Source: CAD feature listing. Evaluate the final solid. Frame: model axes, mm. Face numbers are marked on the shaded views. A direction names the side the tool comes from. Coordinates: 2 decimals unless noted, no trailing zeros. Order: outer loops, then holes, each group sorted by start corner. A loop starts at its lowest first (then second) coordinate and runs counter-clockwise, first axis right, second up.
```python
from build123d import *

# Parameters (mm, degrees)
SKETCH_1_W          = 15
SKETCH_1_H          = 10
EXTRUDE_1_DEPTH     = 5
SKETCH_1_3_W        = 15
SKETCH_1_3_H        = 10
EXTRUDE_2_DEPTH     = 15
CUT_EXTRUDE_1_DEPTH = 15


with BuildPart() as part:
    # Sketch 1 → Extrude 1 (new body)
    with BuildSketch(Plane(origin=(0, 0, 0), x_dir=(1, 0, 0), z_dir=(0, 1, 0))):
        Polygon((-5, -10), (0, -10), (15, 10), (0, 10), (0, 0), (-15, 0), (-15, -5), (-5, -5), align=None)
        with Locations((-7.5, 5)):
            Rectangle(SKETCH_1_W, SKETCH_1_H)
    extrude(amount=EXTRUDE_1_DEPTH)

    # Sketch 1_3 → Extrude 2 (add)
    with BuildSketch(Plane(origin=(0, 0, 0), x_dir=(1, 0, 0), z_dir=(0, 1, 0))):
        with Locations((-7.5, 5)):
            Rectangle(SKETCH_1_3_W, SKETCH_1_3_H)
    extrude(amount=EXTRUDE_2_DEPTH)

    # Sketch 2 → Cut-Extrude 1 (cut)
    with BuildSketch(Plane(origin=(0, 0, 0), x_dir=(0, 0, -1), z_dir=(1, 0, 0))):
        Polygon((10, 15), (0, 10), (0, 15), align=None)
    extrude(amount=-CUT_EXTRUDE_1_DEPTH, mode=Mode.SUBTRACT)


solid = part.part
```
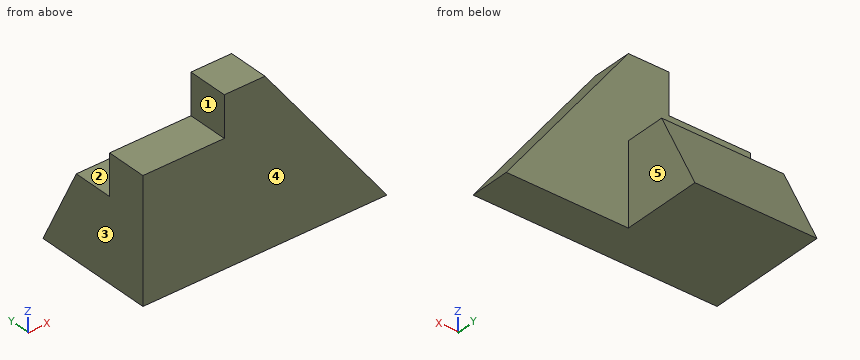
1. Ray query, line 1 (Y direction, x = 3.25, z = -1.25); line 2 (Z direction, x = -8.25, y = 2.75); line 3 (X direction, y = 8.25, z = -5). Return the intervals inside material, ascending.
Findings:
line 1: y = 0 to 5
line 2: z = -10 to 5
line 3: x = -15 to 0
2. Section query D-D on z = 4.5. Return loops of the section in (x, y) (3 decimals), plus the area to 3 significant figures.
Findings:
outline: (-15, 0) - (4.125, 0) - (4.125, 5) - (-15, 5) - close
area: 95.6 mm2
3. Section query A-A on x = -0.75. Return loops of the section in (y, z).
Findings:
outline: (0, -10) - (15, -10) - (10, 0) - (5, 0) - (5, 10) - (0, 10) - close
4. Section query B-B on y = 1.5. Return loops of the section in (x, z).
Findings:
outline: (-15, -10) - (15, -10) - (0, 10) - (-5, 10) - (-5, 5) - (-15, 5) - close
5. Section query C-C on y = 8.75. Return loops of the section in (x, z).
Findings:
outline: (-15, -10) - (0, -10) - (0, 0) - (-15, 0) - close
6. Access query for the marked faces 1, 2, 3, 4 and 5. Directions: +Z, -Z, +X, -X, +Y, -Y. A direction counts if a zero-diameter tool reaches every point of the face in a straight line with its end or side. Return the directions, or none.
Findings:
face 1: +Z, -X, +Y, -Y
face 2: +Z, +X, -X, +Y
face 3: +Z, -Z, -X, +Y, -Y
face 4: +Z, -Z, +X, -X, -Y
face 5: +Z, -Z, +X, +Y
7. Pin query (flat end, axial travel): P1, Ø10, axis at x = 0.5, z = 2, coming from the +Y side; P2, Ø1.5, axis at x = -2.5, z = 3.5, coming from the +Y side; P3, Ø2.5, axis at x = -7.5, y = 7.5, coming from the +Z side; P4, Ø1.5, axis at x = 11, y = 7, coming from the -Z side. Return the tip coordinate at first contact, or that it passes through.
Findings:
P1: stops at y = 11.49
P2: stops at y = 5
P3: stops at z = 0
P4: passes through
